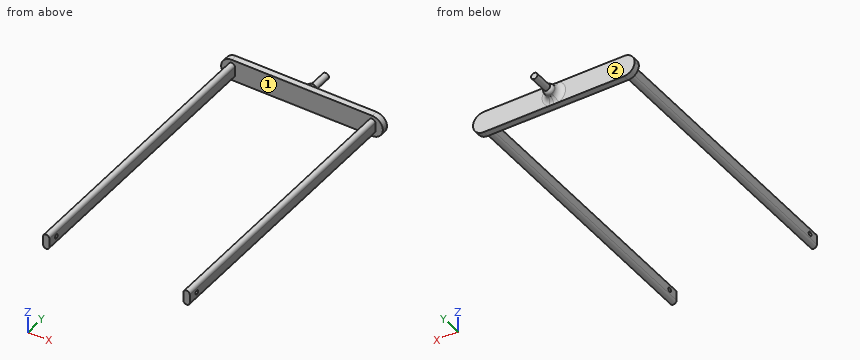
```python
from build123d import *

# Parameters (mm, degrees)
SALIENTE_EXTRUIR1_DEPTH = 3
CROQUIS2_R              = 2.5
SALIENTE_EXTRUIR2_DEPTH = 5
CROQUIS3_R              = 1.5
SALIENTE_EXTRUIR3_DEPTH = 9
REDONDEO1_R             = 2
REDONDEO2_R             = 3
REDONDEO3_R             = 5
SALIENTE_EXTRUIR6_DEPTH = 133
CROQUIS7_R              = 1
CORTAR_EXTRUIR6_DEPTH   = 140


# Some blends are built 0.0001 mm under size
with BuildPart() as part:
    # Croquis1 → Saliente-Extruir1 (new body)
    with BuildSketch(Plane(origin=(0, 0, 0), x_dir=(1, 0, 0), z_dir=(0, 1, 0))):
        Polygon((-38, 0), (-38, 5), (0, 5), (38, 5), (38, 0), (38, -5), (0, -5), (-38, -5), align=None)
    extrude(amount=SALIENTE_EXTRUIR1_DEPTH)

    # Croquis2 → Saliente-Extruir2 (add)
    with BuildSketch(Plane(origin=(0, 3, 0), x_dir=(1, 0, 0), z_dir=(0, 1, 0))):
        with Locations(Location((0, 0, 0), (0, 0, 90))):
            Circle(CROQUIS2_R)
    extrude(amount=SALIENTE_EXTRUIR2_DEPTH)

    # Croquis3 → Saliente-Extruir3 (add)
    with BuildSketch(Plane(origin=(0, 8, 0), x_dir=(1, 0, 0), z_dir=(0, 1, 0))):
        with Locations(Location((0, 0, 0), (0, 0, 270))):
            Circle(CROQUIS3_R)
    extrude(amount=SALIENTE_EXTRUIR3_DEPTH)

    # Redondeo1
    # the kernel refuses this fillet: 2 mm, written as the material it takes off along each edge
    with BuildSketch(Plane(origin=(0, 8, 0), x_dir=(0, 0, -1), z_dir=(1, 0, 0))) as redondeo1_piece_1:
        with BuildLine():
            CenterArc((0.5, -1.732050808), REDONDEO1_R, 0, 60)
            Line((1.5, 0), (1.52, 0.034641016))
            ThreePointArc((1.52, 0.034641016), (2, 0.04), (2.5, 0.04))
            Line((2.5, 0.04), (2.54, 0))
            Line((2.54, 0), (2.54, -1.732050808))
            Line((2.54, -1.732050808), (2.5, -1.732050808))
        make_face()
    revolve(axis=Axis((0, 8, 0), (0, 1, 0)), mode=Mode.SUBTRACT)

    # Redondeo2
    redondeo2_edges = [part.edges().sort_by_distance(p)[0] for p in [
        (0, 3, 2.5),
    ]]
    fillet(redondeo2_edges, radius=REDONDEO2_R)

    # Redondeo3
    redondeo3_edges = [part.edges().sort_by_distance(p)[0] for p in [
        (38, 1.5, 5),
        (38, 1.5, -5),
        (-38, 1.5, -5),
        (-38, 1.5, 5),
    ]]
    fillet(redondeo3_edges, radius=REDONDEO3_R - 0.0001)  # a hair under: the kernel refuses the full size

    # Croquis4 → Saliente-Extruir6 (add)
    with BuildSketch(Plane.XZ):
        with BuildLine():
            Line((-31.5, 2), (-31.5, 0))
            Line((-31.5, 0), (-31.5, -2))
            ThreePointArc((-31.5, -2), (-33, -3.5), (-34.5, -2))
            Line((-34.5, -2), (-34.5, 2))
            ThreePointArc((-34.5, 2), (-33, 3.5), (-31.5, 2))
        make_face()
        with BuildLine():
            Line((31.5, 0), (31.5, -2))
            ThreePointArc((31.5, -2), (33, -3.5), (34.5, -2))
            Line((34.5, -2), (34.5, 2))
            ThreePointArc((34.5, 2), (33, 3.5), (31.5, 2))
            Line((31.5, 2), (31.5, 0))
        make_face()
    extrude(amount=SALIENTE_EXTRUIR6_DEPTH)

    # Croquis7 → Cortar-Extruir6 (cut)
    with BuildSketch(Plane.ZY.offset(34.5)):
        with Locations((0, -128)):
            Circle(CROQUIS7_R)
    extrude(amount=-CORTAR_EXTRUIR6_DEPTH, mode=Mode.SUBTRACT)


solid = part.part
```
Can you work these out from the model? Positions are in its coordinate system, mm. Face numbers are marked on the shaded views. Coordinates: 2 decimals unless noted, no trailing zeros. Write each loop counter-clockwise with the first axis right and the second up, starting at its lowest first coordinate (ties: lowest second). Pieces come first, ordered by that corner, then holes. Notation, with made-up numbers: M -26.75,16.25 L -4.75,16.25 A19 ccw -4.75,50.25 Z; hole C 22,26.25 d4. An arc over 180 degrees is marked long. Answer as CSV lines item,"result".
Item 1: Imagine slicing it at B-B on x = -28. List the corners of the cut face in (y, z) for me.
Geometry results:
outline,"M 0,-5 L 3,-5 L 3,5 L 0,5 Z"
Item 2: Imagine slicing it at A-A on y = -102. List the corners of the cut face in (x, z) for me.
Geometry results:
outline,"M -34.5,-2 A1.5 ccw -31.5,-2 L -31.5,2 A1.5 ccw -34.5,2 Z; M 31.5,-2 A1.5 ccw 34.5,-2 L 34.5,2 A1.5 ccw 31.5,2 Z"
Item 3: Please list where these lines run through material, in increasing order: line 1 along Y through (x, z) = (33.15, 0); line 2 along X through (y, z) = (-88, -1.75); line 3 along Z through (x, y) = (33, -128).
Geometry results:
line 1,"y = -133 to -129, -127 to 3"
line 2,"x = -34.5 to -31.5, 31.5 to 34.5"
line 3,"z = -3.5 to -1, 1 to 3.5"
Item 4: We'd pull the mould along X, two halves only. Please class the marked faces 1 and 2: +X half, -X half, draft (parallel to the pull), parting line (faces both ways), or undercut.
Geometry results:
face 1,"undercut"
face 2,"draft"
Item 5: I'm going to push flat-ended pins straight in: P1, Ø5, axis at x = -16, z = 1.5, coming from the +Y side; P2, Ø1.2, axis at y = -72.5, z = 0, coming from the +X side; P3, Ø3, axis at y = -56.5, z = 1, coming from the -X side; P4, Ø1.8, axis at y = -128, z = 0, coming from the +X side. Where does each tip first touch, or does it pass through?
Geometry results:
P1,"stops at y = 3"
P2,"stops at x = 34.5"
P3,"stops at x = -34.5"
P4,"passes through"
